Design review of the part built by this model. Coordinates are the model's own, in mm. Face numbers are marked on the shaded views. A direction names the side the tool comes from. Coordinates: 2 decimals unless noted, no trailing zeros. Write each loop counter-clockwise with the first axis right and the second up, starting at its lowest first coordinate (ties: lowest second). Pieces come first, ordered by that corner, then holes. Notation, with made-up numbers: (86, -40) - (129, -40) arc R23 cw to (129, -16) - close; hole circle Ø4 at (-25.75, 68.5). An arc over 180 degrees is marked (long way). Answer as CSV lines item,"result". Start each with the question number.
Q1. Machinability: for the marked faces 1 and 2, which of the approach directions +Z, -Z, +X, -X, +Y, -Y give a long, thin tool a straight path to every point of the face, cutting with its end or side? Answer none if there is none.
Q2. We need section B-B (z = -26.5). Write out the cut boundary in (x, y).
Q3. We need section A-A (x = 70). Write out the cut boundary in (y, z).
Q4. We need section D-D (x = -42). Write out the cut boundary in (y, z).
Q5. We need section C-C (y = 0). Write out the cut boundary in (x, z), plus the area to 3 significant figures.
Q6. For line 1 along Y through (x, z) = (-22.5, 0); line 2 along X through (y, z) = (-8, -11); line 3 along Y through (x, z) = (30, -43.25), list the stretches that pass through material, from the lowest coordinate up. Write a range as [from, to].
Q7. Mouldability with a two-part tool opening along X and no side actions: class the marked faces 3, 4 and 5 as pulls with the +X half, pulls with the -X half, needs draft (parallel to the pull), parting line crosses it, or undercut.
Q8. Clearance check with flat-ended pins moving along their axes: pin 1 (6.5 mm diameter, centred on x = 34.5, z = -45.5, fed in from -Y); pin 2 (4 mm diameter, centred on x = -22, z = -14, fed in from +Y); pin 3 (1 mm diameter, centred on x = 58.5, y = 16, fed in from +Z); pin 4 (6.5 mm diameter, centred on y = 0, z = 0, fed in from +X). State where each tip first meets the part, or that it passes through.
from build123d import *

# Parameters (mm, degrees)
SK_SOLE_PLATE_R    = 10
SK_SOLE_PLATE_R_2  = 8
SOLE_PLATE_DEPTH   = 8
SK_CLEVIS_FRONT_R  = 4
CLEVIS_FRONT_DEPTH = 8
SK_CLEVIS_BACK_R   = 4
CLEVIS_BACK_DEPTH  = 8
SK_POST_LAT_W      = 14
SK_POST_LAT_H      = 14
POST_LAT_DEPTH     = 38
SK_POST_MED_W      = 14
SK_POST_MED_H      = 14
POST_MED_DEPTH     = 38


with BuildPart() as part:
    # SK_Sole_Plate → Sole_Plate (new body)
    with BuildSketch(Plane.XY.offset(-50)):
        Polygon((-60, 47.5), (107, 47.5), (135, 25.5), (135, -25.5), (107, -47.5), (-60, -47.5), (-75, -32.5), (-75, 32.5), align=None)
        with Locations((70, 0)):
            Circle(SK_SOLE_PLATE_R, mode=Mode.SUBTRACT)
        with Locations((30, 0)):
            Circle(SK_SOLE_PLATE_R_2, mode=Mode.SUBTRACT)
    extrude(amount=SOLE_PLATE_DEPTH)

    # SK_Clevis_Front → Clevis_Front (add)
    with BuildSketch(Plane(origin=(17.5, 0, 0), x_dir=(0, 0, -1), z_dir=(1, 0, 0))):
        Polygon((42, 13), (42, -13), (-3, -13), (-10, -8), (-10, 8), (-3, 13), align=None)
        Circle(SK_CLEVIS_FRONT_R, mode=Mode.SUBTRACT)
    extrude(amount=CLEVIS_FRONT_DEPTH)

    # SK_Clevis_Back → Clevis_Back (add)
    with BuildSketch(Plane(origin=(-25.5, 0, 0), x_dir=(0, 0, -1), z_dir=(1, 0, 0))):
        Polygon((42, 13), (42, -13), (-3, -13), (-10, -8), (-10, 8), (-3, 13), align=None)
        Circle(SK_CLEVIS_BACK_R, mode=Mode.SUBTRACT)
    extrude(amount=CLEVIS_BACK_DEPTH)

    # SK_Post_Lat → Post_Lat (add)
    with BuildSketch(Plane.XY.offset(-42)):
        with Locations((-40, -45)):
            Rectangle(SK_POST_LAT_W, SK_POST_LAT_H)
    extrude(amount=POST_LAT_DEPTH)

    # SK_Post_Med → Post_Med (add)
    with BuildSketch(Plane.XY.offset(-42)):
        with Locations((-40, 45)):
            Rectangle(SK_POST_MED_W, SK_POST_MED_H)
    extrude(amount=POST_MED_DEPTH)


solid = part.part
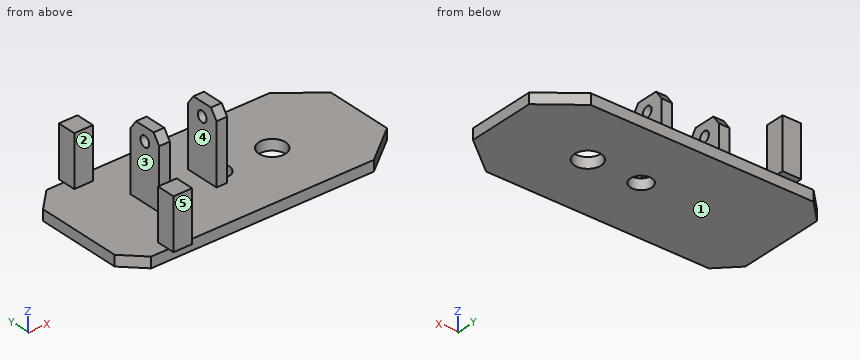
Results list:
1,face 1,"-Z, +X, -X, +Y, -Y"
1,face 2,"+Z, +X, -X"
2,outline,"(-47, -52) - (-33, -52) - (-33, -38) - (-47, -38) - close; (-47, 38) - (-33, 38) - (-33, 52) - (-47, 52) - close; (-25.5, -13) - (-17.5, -13) - (-17.5, 13) - (-25.5, 13) - close; (17.5, -13) - (25.5, -13) - (25.5, 13) - (17.5, 13) - close"
3,outline,"(-47.5, -50) - (-10, -50) - (-10, -42) - (-47.5, -42) - close; (10, -50) - (47.5, -50) - (47.5, -42) - (10, -42) - close"
4,outline,"(-52, -42) - (-47.5, -42) - (-47.5, -50) - (47.5, -50) - (47.5, -42) - (52, -42) - (52, -4) - (38, -4) - (38, -42) - (-38, -42) - (-38, -4) - (-52, -4) - close"
5,outline,"(-75, -50) - (22, -50) - (22, -42) - (25.5, -42) - (25.5, -4) - (17.5, -4) - (17.5, -42) - (-17.5, -42) - (-17.5, -4) - (-25.5, -4) - (-25.5, -42) - (-75, -42) - close; (-25.5, 4) - (-17.5, 4) - (-17.5, 10) - (-25.5, 10) - close; (17.5, 4) - (25.5, 4) - (25.5, 10) - (17.5, 10) - close; (38, -50) - (60, -50) - (60, -42) - (38, -42) - close; (80, -50) - (135, -50) - (135, -42) - (80, -42) - close"
5,area,"2,100 mm2"
6,line 1,"y = [-13, -4], [4, 13]"
6,line 2,"x = [-25.5, -17.5], [17.5, 25.5]"
6,line 3,"y = [-47.5, -8], [8, 47.5]"
7,face 3,"pulls with the -X half"
7,face 4,"undercut"
7,face 5,"needs draft"
8,pin 1,"stops at y = -47.5"
8,pin 2,"stops at y = 13"
8,pin 3,"stops at z = -42"
8,pin 4,"passes through"
